```python
from build123d import *

# Parameters (mm, degrees)
F1_DEPTH = 2
F2_SIZE2 = 0.8660254038
F2_SIZE  = 1.5
F3_W     = 0.5
F3_H     = 5
F3_H_2   = 2.9487536475
F4_DEPTH = 1


with BuildPart() as f1:
    # F0 (on Top) → F1 (new body)
    with BuildSketch(Plane.XY):
        Polygon((-50, -2.5), (50, -2.5), (50, 2.5), (48.5, 2.5), (46.5, 2.5), (43.5, 2.5), (41.5, 2.5), (38.5, 2.5), (36.5, 2.5), (33.5, 2.5), (31.5, 2.5), (28.5, 2.5), (26.5, 2.5), (23.5, 2.5), (21.5, 2.5), (18.5, 2.5), (16.5, 2.5), (13.5, 2.5), (11.5, 2.5), (8.5, 2.5), (6.5, 2.5), (3.5, 2.5), (1.5, 2.5), (-1.5, 2.5), (-3.5, 2.5), (-6.5, 2.5), (-8.5, 2.5), (-11.5, 2.5), (-13.5, 2.5), (-16.5, 2.5), (-18.5, 2.5), (-21.5, 2.5), (-23.5, 2.5), (-26.5, 2.5), (-28.5, 2.5), (-31.5, 2.5), (-33.5, 2.5), (-36.5, 2.5), (-38.5, 2.5), (-40, 2.5), (-41.5, 2.5), (-43.5, 2.5), (-46.5, 2.5), (-48.5, 2.5), (-50, 2.5), align=None)
        Polygon((48.5, 2.5), (50, 2.5), (50, 7.5), align=None)
        Polygon((-50, 7.5), (-50, 2.5), (-48.5, 2.5), align=None)
        Polygon((43.5, 2.5), (46.5, 2.5), (45, 4.5), align=None)
        Polygon((-45, 4.5), (-46.5, 2.5), (-43.5, 2.5), align=None)
        Polygon((38.5, 2.5), (41.5, 2.5), (40, 7.5), align=None)
        Polygon((-40, 7.5), (-41.5, 2.5), (-40, 2.5), (-38.5, 2.5), align=None)
        Polygon((33.5, 2.5), (36.5, 2.5), (35, 4.5), align=None)
        Polygon((-35, 4.5), (-36.5, 2.5), (-33.5, 2.5), align=None)
        Polygon((28.5, 2.5), (31.5, 2.5), (30, 7.5), align=None)
        Polygon((-30, 7.5), (-31.5, 2.5), (-28.5, 2.5), align=None)
        Polygon((23.5, 2.5), (26.5, 2.5), (25, 4.5), align=None)
        Polygon((-25, 4.5), (-26.5, 2.5), (-23.5, 2.5), align=None)
        Polygon((18.5, 2.5), (21.5, 2.5), (20, 7.5), align=None)
        Polygon((-20, 7.5), (-21.5, 2.5), (-18.5, 2.5), align=None)
        Polygon((13.5, 2.5), (16.5, 2.5), (15, 4.5), align=None)
        Polygon((-15, 4.5), (-16.5, 2.5), (-13.5, 2.5), align=None)
        Polygon((8.5, 2.5), (11.5, 2.5), (10, 7.5), align=None)
        Polygon((-10, 7.5), (-11.5, 2.5), (-8.5, 2.5), align=None)
        Polygon((3.5, 2.5), (6.5, 2.5), (5, 4.5), align=None)
        Polygon((-5, 4.5), (-6.5, 2.5), (-3.5, 2.5), align=None)
        Polygon((-1.5, 2.5), (1.5, 2.5), (0, 7.5), align=None)
    extrude(amount=F1_DEPTH)

    # F2
    f2_edges = [f1.edges().sort_by_distance(p)[0] for p in [
        (0, -2.5, 0),
    ]]
    f2_side = f1.faces().sort_by_distance((0, 0.673554, 0))[0]
    chamfer(f2_edges, length=F2_SIZE, length2=F2_SIZE2, reference=f2_side)

    # F3 (on face) → F4 (cut)
    with BuildSketch(Plane.XY.offset(2)):
        with Locations((-40, 0)):
            Rectangle(F3_W, F3_H)
        with Locations((-30, 0)):
            Rectangle(F3_W, F3_H)
        with Locations((-20, 0)):
            Rectangle(F3_W, F3_H)
        with Locations((-10, 0)):
            Rectangle(F3_W, F3_H)
        Rectangle(F3_W, F3_H)
        with Locations((10, 0)):
            Rectangle(F3_W, F3_H)
        with Locations((20, 0)):
            Rectangle(F3_W, F3_H)
        with Locations((30, 0)):
            Rectangle(F3_W, F3_H)
        with Locations((40, 0)):
            Rectangle(F3_W, F3_H)
        with Locations((-45, -1.0256231762)):
            Rectangle(F3_W, F3_H_2)
        with Locations((-35, -1.0256231762)):
            Rectangle(F3_W, F3_H_2)
        with Locations((-25, -1.0256231762)):
            Rectangle(F3_W, F3_H_2)
        with Locations((-15, -1.0256231762)):
            Rectangle(F3_W, F3_H_2)
        with Locations((-5, -1.0256231762)):
            Rectangle(F3_W, F3_H_2)
        with Locations((5, -1.0256231762)):
            Rectangle(F3_W, F3_H_2)
        with Locations((15, -1.0256231762)):
            Rectangle(F3_W, F3_H_2)
        with Locations((25, -1.0256231762)):
            Rectangle(F3_W, F3_H_2)
        with Locations((35, -1.0256231762)):
            Rectangle(F3_W, F3_H_2)
        with Locations((45, -1.0256231762)):
            Rectangle(F3_W, F3_H_2)
    extrude(amount=-F4_DEPTH, mode=Mode.SUBTRACT)


solid = f1.part
```
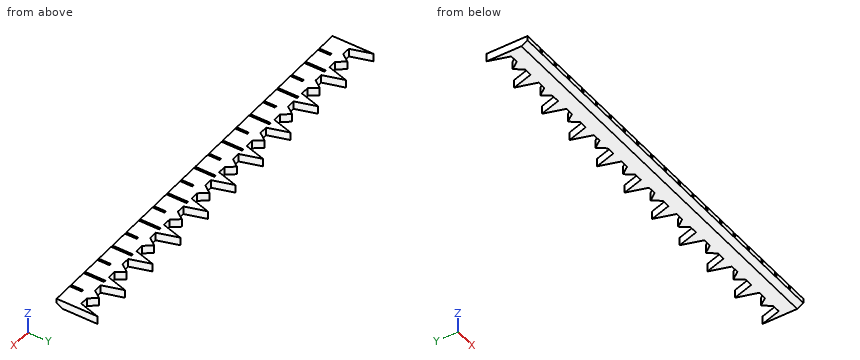
Here's how the part is built. I have some questions about the finished solid (model axes, mm). Coordinates: 2 decimals unless noted, no trailing zeros. Order: outer loops, then holes, each group sorted by start corner. A loop starts at its lowest first (then second) coordinate and runs counter-clockwise, first axis right, second up. Notation, with made-up numbers: M 49,47.25 L 98,47.25 A31 ccw 98,81.25 Z; hole C 1.5,30.25 d10. An arc over 180 degrees is marked long. Answer as a JSON object with one key per item and string values. Group by question number.
(1) Suppose I cut it at A-A, the plane y = 5.5. State how many separate pieces and enclosed holes the cut face has, then the cut area to 3 significant figures.
(2) Suppose I cut it at B-B, the plane x = 7.5. Please give me the cut outline in (y, z).
(3) I need wall thicknesses on probe 1 along Y at (x, z) = (2, 1.45); probe 2 along Y at (x, z) = (-34.5, 1.7). Which ranges of each line are inside material? Lowest first, please.
(4) For pin 1 (1 mm diameter, centred on x = -26.5, z = 0.5, fed in from +Y); pin 2 (0.6 mm diameter, centred on x = 25, y = -0.5, fed in from +Z); pin 3 (0.6 mm diameter, centred on x = -3, z = 1, fed in from +Y), each with a flat end and sliding along its axis, tell me the tip position at first contact or that it passes through.
Values found:
{
 "1": {"separate pieces": "11", "enclosed holes": "0", "area": "24.0 mm^2"},
 "2": {"outline": "M -2.5,0.87 L -1,0 L 2.5,0 L 2.5,2 L -2.5,2 Z"},
 "3": {"probe 1": "y = -2.5 to 2.5", "probe 2": "y = -2.5 to 3.83"},
 "4": {"pin 1": "stops at y = 3.17", "pin 2": "stops at z = 2", "pin 3": "stops at y = 2.5"}
}
